from build123d import *

# Parameters (mm, degrees)
SKETCH_1_R          = 70
SKETCH_1_R_2        = 40
EXTRUDE_1_DEPTH     = 10
SKETCH_2_W          = 120.331390639
SKETCH_2_H          = 328.028138093
CUT_EXTRUDE_1_DEPTH = 62
SKETCH_3_R          = 10.1
CUT_EXTRUDE_2_DEPTH = 2
FILLET_1_R          = 10
SKETCH_4_R          = 2.1
CUT_EXTRUDE_3_DEPTH = 10


with BuildPart() as part:
    # 草图1 → 凸台-拉伸1 (new body)
    with BuildSketch(Plane(origin=(0, 0, 0), x_dir=(1, 0, 0), z_dir=(0, 1, 0))):
        with Locations(Location((0, 0, 0), (0, 0, 270))):
            Circle(SKETCH_1_R)
        with Locations(Location((0, 0, 0), (0, 0, 270))):
            Circle(SKETCH_1_R_2, mode=Mode.SUBTRACT)
    extrude(amount=EXTRUDE_1_DEPTH)

    # 草图2 → 切除-拉伸1 (cut)
    with BuildSketch(Plane(origin=(0, 10, 0), x_dir=(1, 0, 0), z_dir=(0, 1, 0))):
        with Locations((60.16569532, 8.487402818)):
            Rectangle(SKETCH_2_W, SKETCH_2_H)
    extrude(amount=-CUT_EXTRUDE_1_DEPTH, mode=Mode.SUBTRACT)

    # 草图3 → 切除-拉伸2 (cut)
    with BuildSketch(Plane(origin=(0, 10, 0), x_dir=(1, 0, 0), z_dir=(0, 1, 0))):
        with Locations(Location((-35.353318533, -42.132444372, 0), (0, 0, 270))):
            Circle(SKETCH_3_R)
    cut_extrude_2 = extrude(amount=-CUT_EXTRUDE_2_DEPTH, mode=Mode.SUBTRACT)

    # 镜向1: 切除-拉伸2 across plane
    add(cut_extrude_2.mirror(Plane.XY), mode=Mode.SUBTRACT)

    # 圆角1
    fillet_1_edges = [part.edges().sort_by_distance(p)[0] for p in [
        (0, 5, 40),
        (0, 5, -40),
        (0, 5, -70),
        (0, 5, 70),
    ]]
    fillet(fillet_1_edges, radius=FILLET_1_R)

    # 草图4 → 切除-拉伸3 (cut)
    with BuildSketch(Plane(origin=(0, 8, 0), x_dir=(1, 0, 0), z_dir=(0, 1, 0))):
        with Locations(Location((-38.391050289, -38.161023243, 0), (0, 0, 270))):
            Circle(SKETCH_4_R)
        with Locations(Location((-30.395101069, -41.487402065, 0), (0, 0, 270))):
            Circle(SKETCH_4_R)
        with Locations(Location((-37.273804241, -46.748907806, 0), (0, 0, 270))):
            Circle(SKETCH_4_R)
    cut_extrude_3 = extrude(amount=-CUT_EXTRUDE_3_DEPTH, mode=Mode.SUBTRACT)

    # 镜向2: 切除-拉伸3 across plane
    add(cut_extrude_3.mirror(Plane.XY), mode=Mode.SUBTRACT)


solid = part.part
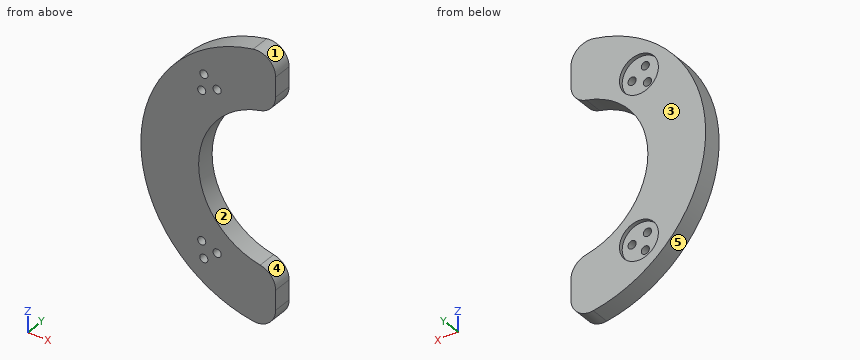
Model file for the job. Use its own axes, mm. Face numbers are marked on the shaded views. A direction names the side the tool comes from. Coordinates: 2 decimals unless noted, no trailing zeros. Order: outer loops, then holes, each group sorted by start corner. A loop starts at its lowest first (then second) coordinate and runs counter-clockwise, first axis right, second up. Notation, with made-up numbers: (79.25, 1) -> (121.25, 1) arc R20 ccw to (121.25, 9) -> close; hole circle Ø1 at (6.25, 21.25). An arc over 180 degrees is marked (long way). Return JSON: item names as keys, results as strings. Group by question number.
Item 1: Saw through at C-C on x = -50. Write the cut outline in (y, z).
Item 2: Saw through at B-B on y = 5.5. Write the cut outline in (x, z), then the cut area to 3 significant figures.
Item 3: Wall check: line 1 along Y through (x, z) = (-36, 38); line 2 along X through (y, z) = (6.5, 48); line 3 along Z through (x, y) = (-7.5, 7.25). Give the ranges that are in metal, low to high. Write a range as [from, to].
Item 4: Saw through at D-D on z = 0. Write the cut outline in (x, y), then the cut area to 3 significant figures.
Item 5: Tool access for the marked faces 4 and 5: list every direction of +Z, -Z, +X, -X, +Y, -Y with a clear straight run to the whole face (end or side of a thin tool).
Item 6: Flat gauge pins, fed straight in: P1, Ø5, axis at x = -60.5, y = 2.5, coming from the +Z side; P2, Ø1.5, axis at x = -54.5, y = 3, coming from the +Z side; P3, Ø5.5, axis at x = -37.27, z = -46.75, coming from the +Y side. Where does each tip first touch, or does it go through?
Item 7: Saw through at A-A on x = -19.5. Write the cut outline in (y, z), then the cut area to 3 significant figures.
Item 8: Pull direction Z, two halves, no side cores. Call the marked faces 1, 2 and 3: pulls with the +Z half, pulls with the -Z half, needs draft (parallel to the pull), parting line crosses it, or undercut.
Values found:
{
 "1": {"outline": "(0, -48.99) -> (10, -48.99) -> (10, 48.99) -> (0, 48.99) -> close"},
 "2": {"outline": "(-11.67, -69.02) arc R10 ccw to (0, -59.16) -> (0, -48.99) arc R10 ccw to (-8, -39.19) arc R40 cw to (-8, 39.19) arc R10 ccw to (0, 48.99) -> (0, 59.16) arc R10 ccw to (-11.67, 69.02) arc R70 ccw to start; hole circle Ø4.2 at (-38.39, -38.16); hole circle Ø4.2 at (-38.39, 38.16); hole circle Ø4.2 at (-37.27, -46.75); hole circle Ø4.2 at (-37.27, 46.75); hole circle Ø4.2 at (-30.4, -41.49); hole circle Ø4.2 at (-30.4, 41.49)", "area": "5,010 mm2"},
 "3": {"line 1": "y = [0, 8]", "line 2": "x = [-50.95, -38.96], [-35.59, -0.05]", "line 3": "z = [-68.84, -39.31], [39.31, 68.84]"},
 "4": {"outline": "(-70, 0) -> (-40, 0) -> (-40, 10) -> (-70, 10) -> close", "area": "300 mm2"},
 "5": {"face 4": "+X, +Y, -Y", "face 5": "-X, +Y, -Y"},
 "6": {"P1": "stops at z = 39.19", "P2": "stops at z = 44.84", "P3": "stops at y = 8"},
 "7": {"outline": "(0, -67.23) -> (10, -67.23) -> (10, -34.92) -> (0, -34.92) -> close; (0, 34.92) -> (10, 34.92) -> (10, 67.23) -> (0, 67.23) -> close", "area": "646 mm2"},
 "8": {"face 1": "pulls with the +Z half", "face 2": "undercut", "face 3": "needs draft"}
}
